Can you work these out from the model? Positions are in its coordinate system, mm. A direction names the side the tool comes from. Give positions to 0.01 mm unless a question says otherwise; leave off trailing zeros. Write each loop counter-clockwise with the first axis right and the second up, starting at its lowest first coordinate (ties: lowest second). Pieces come first, ordered by that corner, then holes.
1. Suppose I cut it at D-D (z = -1). Please give me the cut outline in (x, y), and give its area (3 significant figures).
2. Thinking about a two-plate mould opening in Z: for faces 6 (the flat face through (0, 1, -12.75)), 7 (the flat face through (0, 1, 12.75)), 8 (the flat face through (0, 0, 0)), which applies, pulls with the +Z half, pulls with the -Z half, needs draft (parallel to the pull), parting line crosses it, or undercut?
3. Suppose I cut it at A-A (y = -2.45). Please give me the cut outline in (x, z).
4. If I drill on probe 1 along Z at (x, y) = (-1.25, -1.9); probe 2 along Y at (x, z) = (3.75, -5.5); probe 3 along X at (y, z) = (-1.95, -9.5), over which ranges is the centre line in solid material (lowest first)?
5. Suppose I cut it at B-B (z = -9.25). Please give me the cut outline in (x, y).
6. Suppose I cut it at C-C (x = 0.5). Please give me the cut outline in (y, z).
7. On a 3-axis mill with a long thin cutter (end or side, diameter ignored), from which of +Z, -Z, +X, -X, +Y, -Y can I reach the whole of each face in a straight line? I mean faces 1 (the flat face through (0, -1, -6)), 2 (the flat face through (0, 2, -2.2)), 3 (the flat face through (2.15, -1, -9)), 4 (the flat face through (-1.2, 2, 0)), 5 (the flat face through (0, -1, -12)). Say none if no direction works.
8. I'm going to push flat-ended pins straight in: pin 1 (0.9 mm diameter, centred on x = 1, y = -1.5, fed in from -Z); pin 2 (0.9 mm diameter, centred on x = 1, y = -1.5, fed in from +Z); pin 3 (0.9 mm diameter, centred on y = -2, z = 7.5, fed in from -X). Where does each tip first touch, or does it pass through?
```python
from build123d import *

# Parameters (mm, degrees)
SK_BOARD_W              = 17.7
SK_BOARD_H              = 25.5
EX_BOARD_DEPTH          = 1.6
SK_SENSOR_W             = 2.4
SK_SENSOR_H             = 4.4
EX_SENSOR_DEPTH         = 1
SK_KEEPOUT_STEMMA_W     = 4.3
SK_KEEPOUT_STEMMA_H     = 6
EX_KEEPOUT_STEMMA_DEPTH = 3


with BuildPart() as part:
    # SK_Board → EX_Board (new body)
    with BuildSketch(Plane(origin=(0, 0, 0), x_dir=(1, 0, 0), z_dir=(0, 1, 0))):
        Rectangle(SK_BOARD_W, SK_BOARD_H)
    extrude(amount=EX_BOARD_DEPTH)

    # SK_Sensor → EX_Sensor (add)
    with BuildSketch(Plane(origin=(0, 1.6, 0), x_dir=(1, 0, 0), z_dir=(0, 1, 0))):
        Rectangle(SK_SENSOR_W, SK_SENSOR_H)
    extrude(amount=EX_SENSOR_DEPTH)

    # SK_KeepOut_STEMMA → EX_KeepOut_STEMMA (add)
    with BuildSketch(Plane(origin=(0, 0, 0), x_dir=(1, 0, 0), z_dir=(0, 1, 0))):
        with Locations((0, -9)):
            Rectangle(SK_KEEPOUT_STEMMA_W, SK_KEEPOUT_STEMMA_H)
        with Locations((0, 9)):
            Rectangle(SK_KEEPOUT_STEMMA_W, SK_KEEPOUT_STEMMA_H)
    extrude(amount=-EX_KEEPOUT_STEMMA_DEPTH)


solid = part.part
```
Checks:
1. outline: (-8.85, 0) - (8.85, 0) - (8.85, 1.6) - (1.2, 1.6) - (1.2, 2.6) - (-1.2, 2.6) - (-1.2, 1.6) - (-8.85, 1.6) - close
1. area: 30.7 mm2
2. face 6: pulls with the -Z half
2. face 7: pulls with the +Z half
2. face 8: undercut
3. outline: (-2.15, -12) - (2.15, -12) - (2.15, -6) - (-2.15, -6) - close; (-2.15, 6) - (2.15, 6) - (2.15, 12) - (-2.15, 12) - close
4. probe 1: z = -12 to -6, 6 to 12
4. probe 2: y = 0 to 1.6
4. probe 3: x = -2.15 to 2.15
5. outline: (-8.85, 0) - (-2.15, 0) - (-2.15, -3) - (2.15, -3) - (2.15, 0) - (8.85, 0) - (8.85, 1.6) - (-8.85, 1.6) - close
6. outline: (-3, -12) - (0, -12) - (0, -12.75) - (1.6, -12.75) - (1.6, -2.2) - (2.6, -2.2) - (2.6, 2.2) - (1.6, 2.2) - (1.6, 12.75) - (0, 12.75) - (0, 12) - (-3, 12) - (-3, 6) - (0, 6) - (0, -6) - (-3, -6) - close
7. face 1: +X, -X, -Y
7. face 2: -Z, +X, -X, +Y
7. face 3: +Z, -Z, +X, -Y
7. face 4: +Z, -Z, -X, +Y
7. face 5: -Z, +X, -X, -Y
8. pin 1: stops at z = -12
8. pin 2: stops at z = 12
8. pin 3: stops at x = -2.15
